Work out the finished part from the listing and answer in its coordinate system (mm). Give positions to 0.01 mm unless a question says otherwise; leave off trailing zeros. Loops run counter-clockwise (first coordinate to the right, second up) from the corner with the lowest first, then second, coordinate; pieces in that order, holes last. Notation, with made-up numbers: M 77,33 L 98,33 A19 ccw 98,61 Z; hole C 46,-33 d5. An arc over 180 degrees is marked long. Answer as a JSON object with one key per item and string values. Group by question number.
Autodesk Inventor part; units mm, degrees
ref_plane "YZ Plane" through (0, 0, 0) normal (1, 0, 0) x (0, 1, 0)
ref_plane "XZ Plane" through (0, 0, 0) normal (0, 1, 0) x (-1, 0, 0)
ref_plane "XY Plane" through (0, 0, 0) normal (0, 0, 1) x (1, 0, 0)
sketch "Sketch1" plane through (0, 0, 0) normal (0, 1, 0) x (-1, 0, 0)
  line L0 (0, 0) -> (230, 0)
  line L1 (230, 0) -> (230, -180)
  line L2 (230, -180) -> (0, -180)
  line L3 (0, -180) -> (0, 0)
  dimension "d0" = 180
  dimension "d1" = 230
extrude "Extrusion1" add sketch "Sketch1" along normal blind 5
sketch "Sketch2" plane through (0, 0, -180) normal (0, 0, -1) x (-1, 0, 0)
  line L0 (0, 5) -> (230, 5)
  line L1 (55, 5) -> (75, 5)
  line L2 (75, 5) -> (75, 0)
  line L3 (75, 0) -> (55, 0)
  line L4 (55, 0) -> (55, 5)
  line L5 (0, 0) -> (230, 0)
  line L6 (155, 5) -> (175, 5)
  line L7 (175, 5) -> (175, 0)
  line L8 (175, 0) -> (155, 0)
  line L9 (155, 0) -> (155, 5)
  line L10 (0, 0) -> (0, 5)
  line L11 (230, 0) -> (230, 5)
  point P0 (175, 2.5)
  point P1 (155, 2.5)
  point P2 (230, 2.5)
  dimension "d4" = 20
  dimension "d5" = 20
  dimension "d6" = 80
  dimension "d7" = 55
  dimension "d8" = 55
extrude "Extrusion2" add sketch "Sketch2" along normal blind 5 and the other way blind 185 contours L0 L2 L3 L4 | L0 L7 L5 L9
sketch "Sketch3" plane through (0, 0, 0) normal (1, 0, 0) x (0, 0, -1)
  line L0 (0, 5) -> (180, 5)
  line L1 (0, 0) -> (180, 0)
  line L2 (75, 5) -> (105, 5)
  line L3 (105, 5) -> (105, 0)
  line L4 (105, 0) -> (75, 0)
  line L5 (75, 0) -> (75, 5)
  line L6 (180, 0) -> (180, 5)
  point P0 (180, 2.5)
  dimension "d13" = 30
  dimension "d14" = 75
extrude "Extrusion3" add sketch "Sketch3" along normal blind 5 and the other way blind 235 contours L0 L3 L1 L5
sketch "Sketch4" plane through (0, 5, 0) normal (0, 1, 0) x (1, 0, 0)
  line L0 (-230, 75) -> (-230, 0)
  line L1 (0, 180) -> (-55, 180)
  point P0 (0, 0)
  point P1 (-211, 160.5)
  point P2 (-19, 160.5)
  point P3 (-19, 19.5)
  point P4 (-211, 19.5)
  point P5 (-230, 37.5)
  dimension "d19" = 141
  dimension "d20" = 192
  dimension "d21" = 19
  dimension "d22" = 141
  dimension "d23" = 0
  dimension "d24" = 19.5
hole "Hole1" at (-211, 5, -160.5) at (-19, 5, -160.5) at (-19, 5, -19.5) at (-211, 5, -19.5) direction (0, -1, 0) diameter 2.459 end through all
properties part number "onderkant"
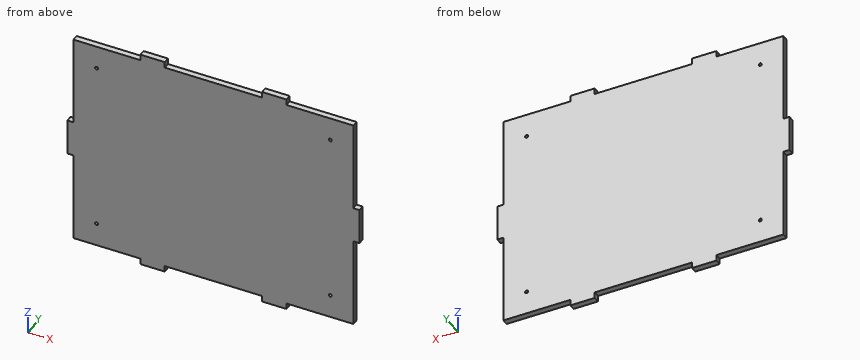
Item 1: A cutting plane is placed at A-A (y = 2.75). Give the number of separate pieces and of enclosed holes in the cut face, and give its area (3 significant figures).
Item 2: Find the intervals of material crossed by probe 1 along X at (y, z) = (2.7, -19.5); probe 2 along Z at (x, y) = (-211, 2.6); probe 3 along Z at (x, y) = (-18, 1.2), in increasing order. Write a range as [from, to].
Item 3: A cutting plane is placed at C-C (z = -140.5). Determine the outline of the cut face in (x, y).
Item 4: A cutting plane is placed at B-B (x = -122). Determine the outline of the cut face in (y, z).
Item 5: Given pin 1 Ø1.5 at (x, y) = (-207, 2) entering from +Z; pin 2 Ø1.5 at (y, z) = (1, -68) entering from +X; pin 3 Ø1.5 at (y, z) = (1.5, -182) entering from -X, each flat-ended and moving along its own axis, determine where each tip first touches the part or whether it passes through.
The answers:
{
 "1": {"separate pieces": "1", "enclosed holes": "4", "area": "42,100 mm^2"},
 "2": {"probe 1": "x = [-230, -212.23], [-209.77, -20.23], [-17.77, 0]", "probe 2": "z = [-180, -161.73], [-159.27, -20.73], [-18.27, 0]", "probe 3": "z = [-180, -161.22], [-159.78, -20.22], [-18.78, 0]"},
 "3": {"outline": "M -230,0 L 0,0 L 0,5 L -230,5 Z"},
 "4": {"outline": "M 0,-180 L 5,-180 L 5,0 L 0,0 Z"},
 "5": {"pin 1": "stops at z = 0", "pin 2": "stops at x = 0", "pin 3": "stops at x = -175"}
}
